Model file for the job. Use its own axes, mm. A direction names the side the tool comes from. Coordinates: 2 decimals unless noted, no trailing zeros. Order: outer loops, then holes, each group sorted by start corner. A loop starts at its lowest first (then second) coordinate and runs counter-clockwise, first axis right, second up.
from build123d import *

# Parameters (mm, degrees)
SKETCH1_R           = 9.575
SKETCH1_R_2         = 7.575
BOSS_EXTRUDE1_DEPTH = 1
BOSS_EXTRUDE2_START = 1.5
SKETCH2_R           = 9.575
BOSS_EXTRUDE2_DEPTH = 1.5
SKETCH3_R           = 2.575
CUT_EXTRUDE1_DEPTH  = 1
CHAMFER1_SIZE       = 0.2
SKETCH4_R           = 0.825
CUT_EXTRUDE2_DEPTH  = 14.623921976


with BuildPart() as part:
    # Sketch1 → Boss-Extrude1 (new body)
    with BuildSketch(Plane(origin=(0, 0, 0), x_dir=(1, 0, 0), z_dir=(0, 1, 0))):
        with Locations(Location((0, 0, 0), (0, 0, 270))):
            Circle(SKETCH1_R)
        with Locations(Location((0, 0, 0), (0, 0, 270))):
            Circle(SKETCH1_R_2, mode=Mode.SUBTRACT)
    extrude(amount=BOSS_EXTRUDE1_DEPTH)

    # Sketch2 → Boss-Extrude2 (add)
    with BuildSketch(Plane.XZ.offset(BOSS_EXTRUDE2_START)):
        with Locations(Location((0, 0, 0), (0, 0, 270))):
            Circle(SKETCH2_R)
    extrude(amount=-BOSS_EXTRUDE2_DEPTH)

    # Sketch3 → Cut-Extrude1 (cut)
    with BuildSketch(Plane.XZ.offset(1.5)):
        with Locations(Location((0, 0, 0), (0, 0, 270))):
            Circle(SKETCH3_R)
    extrude(amount=-CUT_EXTRUDE1_DEPTH, mode=Mode.SUBTRACT)

    # Chamfer1
    chamfer1_edges = [part.edges().sort_by_distance(p)[0] for p in [
        (0, -1.5, 2.575),
    ]]
    chamfer(chamfer1_edges, length=CHAMFER1_SIZE)

    # Sketch4 → Cut-Extrude2 (cut, through all)
    with BuildSketch(Plane.XZ.offset(0.5)):
        with Locations(Location((0, 0, 0), (0, 0, 270))):
            Circle(SKETCH4_R)
    extrude(amount=-CUT_EXTRUDE2_DEPTH, mode=Mode.SUBTRACT)


solid = part.part
Q1. Drop flat-ended pins along their axis: P1, Ø4.5, axis at x = -3.5, z = -1, coming from the +Y side; P2, Ø1.5, axis at x = 0, z = 0, coming from the +Y side; P3, Ø1.5, axis at x = -1, z = 0.5, coming from the -Y side; P4, Ø1, axis at y = -1, z = -1.5, coming from the -X side. Give the stop position or say it passes through.
Established:
P1: stops at y = 0
P2: passes through
P3: stops at y = -0.5
P4: stops at x = -9.52
Q2. Which spindle directions (+Z, -Z, +X, -X, +Y, -Y) get a long thin tool onto all of the face, cutting with end or side? Do faces 1 (the face through (-2.514, -0.906, 0.558)), 2 (the face through (2.3, -1.5, -2)), 3 (the face through (-7.395, 0.493, -1.642)). Say none if no direction does.
Established:
face 1: -Y
face 2: +Z, -Z, +X, -X, -Y
face 3: +Y
Q3. Probe line 1 (X direction, y = -0.4, z = 0) (3 decimals); line 2 (X direction, y = -1.1, z = 0) (3 decimals); line 3 (Y direction, x = 6.5, z = 3). List the from-to ranges inside material, lowest first.
Established:
line 1: x = -9.575 to -0.825, 0.825 to 9.575
line 2: x = -9.575 to -2.575, 2.575 to 9.575
line 3: y = -1.5 to 0
Q4. Cut at D-D, the plane z = -6.5. List the corners of the cut face in (x, y), plus the area to 3 significant figures.
Established:
outline: (-7.03, -1.5) - (7.03, -1.5) - (7.03, 1) - (3.89, 1) - (3.89, 0) - (-3.89, 0) - (-3.89, 1) - (-7.03, 1) - close
area: 27.4 mm2
Q5. Mould opens along Z. For faces 4 (the face through (-2, 0, 0)), 5 (the face through (8, 1, 1)), 6 (the face through (1, -0.5, 1)) say: pulls with the +Z half, pulls with the -Z half, needs draft (parallel to the pull), parting line crosses it, or undercut.
Established:
face 4: undercut
face 5: needs draft
face 6: undercut
Q6. Cut at C-C, the plane x = -5. List the corners of the cut face in (y, z).
Established:
outline: (-1.5, -8.17) - (1, -8.17) - (1, -5.69) - (0, -5.69) - (0, 5.69) - (1, 5.69) - (1, 8.17) - (-1.5, 8.17) - close
Q7. Cut at B-B, the plane x = 0. List the corners of the cut face in (y, z) (3 decimals), plus the area to 3 significant figures.
Established:
outline: (-1.5, -9.575) - (1, -9.575) - (1, -7.575) - (0, -7.575) - (0, -0.825) - (-0.5, -0.825) - (-0.5, -2.575) - (-1.3, -2.575) - (-1.5, -2.775) - close; (-1.5, 2.775) - (-1.3, 2.575) - (-0.5, 2.575) - (-0.5, 0.825) - (0, 0.825) - (0, 7.575) - (1, 7.575) - (1, 9.575) - (-1.5, 9.575) - close
area: 26.7 mm2
Q8. Cut at A-A, the plane z = 0. List the corners of the cut face in (x, y) (3 decimals).
Established:
outline: (-9.575, -1.5) - (-2.775, -1.5) - (-2.575, -1.3) - (-2.575, -0.5) - (-0.825, -0.5) - (-0.825, 0) - (-7.575, 0) - (-7.575, 1) - (-9.575, 1) - close; (0.825, -0.5) - (2.575, -0.5) - (2.575, -1.3) - (2.775, -1.5) - (9.575, -1.5) - (9.575, 1) - (7.575, 1) - (7.575, 0) - (0.825, 0) - close
